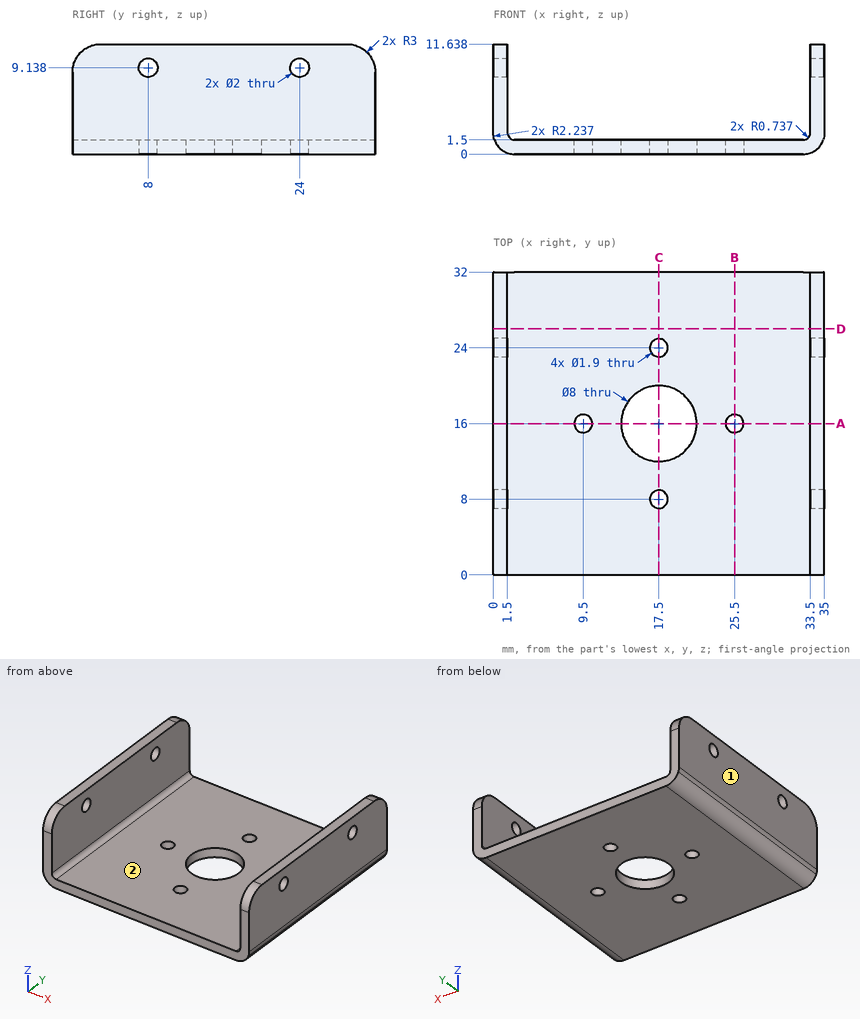
Geometry check sheet. Reference: drawing and pictorial views, mm from the part's lowest x, y, z. A direction names the side the tool comes from. Coordinates: 2 decimals unless noted, no trailing zeros. Loops run counter-clockwise (first coordinate to the right, second up) from the corner with the lowest first, then second, coordinate; pieces in that order, holes last.
1) Sectioned sample at C-C (x = 17.5). Record the boundary of the cut face in (y, z), and give its area (3 significant figures).
2) Sectioned sample at B-B (x = 25.5). Record the boundary of the cut face in (y, z).
3) Sectioned sample at A-A (y = 16). Count the separate pieces of the cut face and the enclosed holes in it.
4) Sectioned sample at D-D (y = 26). Record the boundary of the cut face in (x, z) (1 decimal).
5) Access from +Z, -Z, +X, -X, +Y, -Y to the whole of each face (thin tool, end or side, straight path). Record for the marked faces 1 and 2.
6) Gauge pin test, flat ends, axial feed: pin 1 (1.5 mm diameter, centred on x = 22, z = 2, fed in from -Y); pin 2 (15.5 mm diameter, centred on x = 14, y = 12, fed in from +Z). Record the tip position at first contact, or that the pin passes through.
7) Material ranges on probe 1 along Y at (x, z) = (17.5, 1); probe 2 along X at (y, z) = (30.5, 9.25); probe 3 along Z at (x, y) = (21, 23), recorded low to high.
Check sheet entries:
1. outline: (0, 0) - (7.05, 0) - (7.05, 1.5) - (0, 1.5) - close; (8.95, 0) - (12, 0) - (12, 1.5) - (8.95, 1.5) - close; (20, 0) - (23.05, 0) - (23.05, 1.5) - (20, 1.5) - close; (24.95, 0) - (32, 0) - (32, 1.5) - (24.95, 1.5) - close
1. area: 30.3 mm2
2. outline: (0, 0) - (15.05, 0) - (15.05, 1.5) - (0, 1.5) - close; (16.95, 0) - (32, 0) - (32, 1.5) - (16.95, 1.5) - close
3. separate pieces: 4
3. enclosed holes: 0
4. outline: (0, 2.2) arc R2.2 ccw to (2.2, 0) - (32.8, 0) arc R2.2 ccw to (35, 2.2) - (35, 11.6) - (33.5, 11.6) - (33.5, 2.2) arc R0.7 cw to (32.8, 1.5) - (2.2, 1.5) arc R0.7 cw to (1.5, 2.2) - (1.5, 11.6) - (0, 11.6) - close
5. face 1: +Z, -Z, -X, +Y, -Y
5. face 2: +Z, +Y, -Y
6. pin 1: stops at y = 0
6. pin 2: stops at z = 1.5
7. probe 1: y = 0 to 7.05, 8.95 to 12, 20 to 23.05, 24.95 to 32
7. probe 2: x = 0 to 1.5, 33.5 to 35
7. probe 3: z = 0 to 1.5
